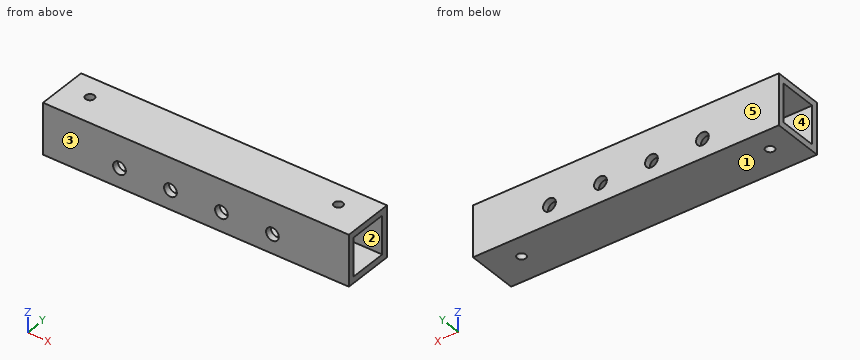
Autodesk Inventor part; units mm, degrees
ref_plane "YZ Plane" through (0, 0, 0) normal (1, 0, 0) x (0, 1, 0)
ref_plane "XZ Plane" through (0, 0, 0) normal (0, 1, 0) x (-1, 0, 0)
ref_plane "XY Plane" through (0, 0, 0) normal (0, 0, 1) x (1, 0, 0)
sketch "Sketch1" plane through (0, 0, 0) normal (1, 0, 0) x (0, 1, 0)
  line L0 (0, 0) -> (25.4, 0)
  line L1 (25.4, 0) -> (25.4, -25.4)
  line L2 (25.4, -25.4) -> (0, -25.4)
  line L3 (0, -25.4) -> (0, 0)
  line L4 (3.175, -3.175) -> (22.225, -3.175)
  line L5 (22.225, -3.175) -> (22.225, -22.225)
  line L6 (22.225, -22.225) -> (3.175, -22.225)
  line L7 (3.175, -22.225) -> (3.175, -3.175)
  dimension "d0" = 25.4
  dimension "d1" = 25.4
  dimension "d2" = 19.05
  dimension "d3" = 19.05
  dimension "d4" = 3.175
  dimension "d5" = 3.175
extrude "Extrusion1" add sketch "Sketch1" along normal blind 152.4
sketch "Sketch2" plane through (0, 25.4, 0) normal (0, 1, 0) x (1, 0, 0)
  line L0 (0, 0) -> (0, 25.4)
  line L1 (0, 0) -> (152.4, 0)
  line L2 (152.4, 25.4) -> (152.4, 0)
  point P0 (38.1, 15.875)
  point P1 (114.3, 15.875)
  dimension "d8" = 38.1
  dimension "d9" = 15.875
  dimension "d10" = 15.875
  dimension "d11" = 38.1
hole "Hole1" at (38.1, 25.4, -15.875) at (114.3, 25.4, -15.875) direction (0, -1, 0) diameter 6.35 end through all
sketch "Sketch3" plane through (0, 0, 0) normal (0, 0, 1) x (1, 0, 0)
  line L0 (0, 0) -> (0, 25.4)
  line L1 (0, 0) -> (152.4, 0)
  line L2 (152.4, 25.4) -> (152.4, 0)
  point P0 (12.7, 14.2875)
  point P1 (136.525, 14.2875)
  dimension "d19" = 15.875
  dimension "d20" = 14.2875
  dimension "d21" = 12.7
  dimension "d22" = 14.2875
hole "Hole2" at (12.7, 14.2875, 0) at (136.525, 14.2875, 0) direction (0, 0, -1) diameter 4.3656 end through all
sketch "Sketch4" plane through (0, 25.4, 0) normal (0, 1, 0) x (1, 0, 0)
  line L0 (0, 0) -> (152.4, 0)
  line L1 (0, 0) -> (0, 25.4)
  point P0 (63.5, 15.875)
  dimension "d30" = 15.875
  dimension "d39" = 63.5
hole "Hole3" at (63.5, 25.4, -15.875) direction (0, -1, 0) diameter 6.35 end through all
sketch "Sketch5" plane through (0, 25.4, 0) normal (0, 1, 0) x (1, 0, 0)
  circle A0 centre (114.3, 15.875) radius 3.175
  line L0 (0, 25.4) -> (152.4, 25.4)
  point P0 (88.9, 15.875)
  dimension "d40" = 9.525
  dimension "d41" = 25.4
hole "Hole4" at (88.9, 25.4, -15.875) direction (0, -1, 0) diameter 6.35 depth 25.4 tip angle 118
properties part number "1x1 pickup arm support rear" material "Aluminum 6061"
The listing builds one solid part. Answer for the finished solid, in the listing's coordinates (mm). Face numbers are marked on the shaded views. A direction names the side the tool comes from. Coordinates: 2 decimals unless noted, no trailing zeros. Write each loop counter-clockwise with the first axis right and the second up, starting at its lowest first coordinate (ties: lowest second). Pieces come first, ordered by that corner, then holes. Notation, with made-up numbers: M 49.5,41 L 101.5,41 A28 cw 101.5,74 Z; hole C 54.25,70.5 d9. An arc over 180 degrees is marked long. Put each result on its own line as item: value. Start each with the question number.
1. A cutting plane is placed at C-C on z = -10.5. Write down the section's boundary in (x, y) (3 decimals), then the cut area to 3 significant figures.
2. For a pull along Y with two mould halves and no side action, classify the marked faces 1, 2 and 3 as pulls with the +Y half, pulls with the -Y half, needs draft (parallel to the pull), parting line crosses it, or undercut.
3. A flat-ended cylindrical pin translates along its axis: P1, Ø2.5, axis at x = 12.7, y = 14.29, coming from the -Z side. Find the tip coordinate at first contact, or state that the pin passes through.
4. Which of the six approach directions +Z, -Z, +X, -X, +Y, -Y give full straight-line access (tool end or side, diameter ignored) to the marked faces 4 and 5?
5. Consider line 1 (Z direction, x = 63.5, y = 1.45); line 2 (Z direction, x = 81, y = 17.5) (3 decimals); line 3 (Y direction, x = 50.5, z = -4.5) (3 decimals). Determine where each line is inside the solid, lowest interval first. Write a range as from..to.
6. A cutting plane is placed at D-D on x = 83. Write down the section's boundary in (y, z) (3 decimals), then the cut area to 3 significant figures.
7. A cutting plane is placed at A-A on x = 12.7. Write down the section's boundary in (y, z) (3 decimals).
8. A cutting plane is placed at B-B on y = 5.5. Write down the section's boundary in (x, z) (3 decimals), then the cut area to 3 significant figures.
Resolved:
1. outline: M 0,0 L 152.4,0 L 152.4,3.175 L 0,3.175 Z; M 0,22.225 L 152.4,22.225 L 152.4,25.4 L 0,25.4 Z
1. area: 968 mm2
2. face 1: needs draft
2. face 2: undercut
2. face 3: pulls with the -Y half
3. P1: passes through
4. face 4: +X, -X
4. face 5: +Z, -Z, +X, -X, +Y
5. line 1: z = -25.4..-19.05, -12.7..0
5. line 2: z = -25.4..-22.225, -3.175..0
5. line 3: y = 0..3.175, 22.225..25.4
6. outline: M 0,-25.4 L 25.4,-25.4 L 25.4,0 L 0,0 Z; hole M 3.175,-22.225 L 22.225,-22.225 L 22.225,-3.175 L 3.175,-3.175 Z
6. area: 282 mm2
7. outline: M 0,-25.4 L 12.105,-25.4 L 12.105,-22.225 L 3.175,-22.225 L 3.175,-3.175 L 12.105,-3.175 L 12.105,0 L 0,0 Z; M 16.47,-25.4 L 25.4,-25.4 L 25.4,0 L 16.47,0 L 16.47,-3.175 L 22.225,-3.175 L 22.225,-22.225 L 16.47,-22.225 Z
8. outline: M 0,-25.4 L 152.4,-25.4 L 152.4,-22.225 L 0,-22.225 Z; M 0,-3.175 L 152.4,-3.175 L 152.4,0 L 0,0 Z
8. area: 968 mm2
